Could you check a few things on this model? Use its own coordinates, in mm. A direction names the side the tool comes from. Coordinates: 2 decimals unless noted, no trailing zeros. Write each loop counter-clockwise with the first axis right and the second up, starting at its lowest first coordinate (ties: lowest second). Pieces come first, ordered by that corner, then holes.
Item 1: I want a section at C-C on x = 3. Please give me the cut outline in (y, z).
Item 2: Thinking about a two-plate mould opening in Z: for faces 1 (the flat face through (-3, 12, 50)), 2 (the flat face through (4, 0, 25)), 3 (the cylindrical face through (3.125, 8.112, 39.538)), which applies, +Z half, -Z half, draft (parallel to the pull), parting line (faces both ways), or undercut?
Item 3: If I drill on probe 1 along Z at (x, y) = (3.75, 13.25); probe 2 along X at (y, z) = (5.75, 13); probe 3 along Z at (x, y) = (6, 1.5), over which ranges is the centre line in solid material (lowest first)?
Item 4: I want a section at D-D on z = 8. Please give me the cut outline in (x, y).
Item 5: For P1, Ø6, axis at y = 6.5, z = 17, coming from the -X side, with a flat end and sliding along its axis, tell me the tip position at first contact or that it passes through.
Item 6: I want a section at A-A on z = 13. Please give me the cut outline in (x, y), then the cut area to 3 significant figures.
Item 7: Which directions (+Z, -Z, +X, -X, +Y, -Y) give clear straight access to the entire face, cutting with the end or side of a thin tool? Please do faces 4 (the cylindrical face through (3.125, 8.112, 15.538)), 5 (the flat face through (0, 5, 25)).
Item 8: I want a section at B-B on y = 12.5. Please give me the cut outline in (x, z).
Autodesk Inventor part; units mm, degrees
ref_plane "YZ Plane" through (0, 0, 0) normal (1, 0, 0) x (0, 1, 0)
ref_plane "XZ Plane" through (0, 0, 0) normal (0, 1, 0) x (-1, 0, 0)
ref_plane "XY Plane" through (0, 0, 0) normal (0, 0, 1) x (1, 0, 0)
sketch "Эскиз1" plane through (0, 0, 0) normal (0, 0, 1) x (1, 0, 0)
  line L0 (0, 0) -> (-20, 0) construction
  line L1 (-20, 0) -> (-20, 10) construction
  line L2 (-20, 10) -> (0, 10) construction
  line L3 (0, 10) -> (0, 0) construction
  line L4 (-20, 0) -> (8.2, 0) construction
  line L5 (8.2, 0) -> (8.2, 16)
  line L6 (8.2, 16) -> (-20, 16)
  line L7 (-20, 16) -> (-20, 0) construction
  line L8 (-20, 16) -> (-20, 10)
  line L9 (-20, 10) -> (0, 10)
  line L10 (0, 10) -> (0, 0)
  line L11 (0, 0) -> (8.2, 0)
  point P0 (-10, 10)
  dimension "d0" = 20
  dimension "d1" = 10
  dimension "d2" = 6
  dimension "d3" = 8.2
extrude "Выдавливание1" add sketch "Эскиз1" along normal blind 50
sketch "Эскиз3" plane through (-20, 16, 0) normal (0, 1, 0) x (1, 0, 0)
  circle A0 centre (23.6882, -13) radius 6 construction
  circle A1 centre (23.6882, -13) radius 2.6
  line L0 (28.2, 0) -> (0, 0)
  circle A2 centre (23.6882, -37) radius 2.6
  line L1 (28.2, -50) -> (0, -50)
  circle A3 centre (23.6882, -13) radius 9 construction
  circle A4 centre (23.6882, -37) radius 9 construction
  circle A5 centre (23.6882, 52.7109) radius 2.5 construction
  circle A6 centre (23.6882, 52.7109) radius 6
  line L2 (17.6882, 52.7109) -> (17.6882, -70.8519) construction
  line L3 (23.6882, -13) -> (23.6882, -47.2953) construction
  line L4 (20, 0) -> (20, -50)
  dimension "d26" = 12
  dimension "d16" = 12
  dimension "d17" = 5.2
  dimension "d20" = 5.2
  dimension "d22" = 24
  dimension "d23" = 18
  dimension "d24" = 18
  dimension "d25" = 13
extrude "Выдавливание4" cut sketch "Эскиз3" against normal blind 20 contours A1 | A2
equation "\"Радиус_гибки\" = Толщина"
equation "\"Ширина_просечки\" = Толщина"
equation "\"Глубина_просечки\" = 0.5 * Толщина"
equation "\"Размер_просечки\" = 4 * Толщина"
equation "\"Мин_остаток\" = 2 * Толщина"
equation "\"Радиус_перехода\" = Радиус_гибки"
equation "\"Радиус_Якоби\" = Радиус_гибки"
equation "\"Размер_зазора\" = Толщина"
properties part number "креп_центр_м2" material "Полипропилен"
Response values:
1. outline: (0, 0) - (16, 0) - (16, 10.49) - (0, 10.49) - close; (0, 15.51) - (16, 15.51) - (16, 34.49) - (0, 34.49) - close; (0, 39.51) - (16, 39.51) - (16, 50) - (0, 50) - close
2. face 1: +Z half
2. face 2: draft
2. face 3: undercut
3. probe 1: z = 0 to 10.4, 15.6 to 34.4, 39.6 to 50
3. probe 2: x = 0 to 1.09, 6.29 to 8.2
3. probe 3: z = 0 to 11.81, 14.19 to 35.81, 38.19 to 50
4. outline: (-20, 10) - (0, 10) - (0, 0) - (8.2, 0) - (8.2, 16) - (-20, 16) - close
5. P1: stops at x = 0
6. outline: (-20, 10) - (0, 10) - (0, 0) - (1.09, 0) - (1.09, 16) - (-20, 16) - close; (6.29, 0) - (8.2, 0) - (8.2, 16) - (6.29, 16) - close
6. area: 168 mm2
7. face 4: +Y, -Y
7. face 5: +Z, -Z, -X, -Y
8. outline: (-20, 0) - (8.2, 0) - (8.2, 50) - (-20, 50) - close; hole circle Ø5.2 at (3.69, 13); hole circle Ø5.2 at (3.69, 37)
